Design review of the part built by this model. Coordinates are the model's own, in mm. A direction names the side the tool comes from. Coordinates: 2 decimals unless noted, no trailing zeros. Loops run counter-clockwise (first coordinate to the right, second up) from the corner with the lowest first, then second, coordinate; pieces in that order, holes last. Notation, with made-up numbers: M -31.5,54.25 L -19.5,54.25 A25 cw -19.5,77.25 Z; hole C 4.5,-23.5 d8. An arc over 180 degrees is marked long. Answer as a JSON object with one key per item and string values. Group by question number.
1. Consider section D-D (x = 10.5). State the section outline as (y, z) points.
2. Consider section A-A (x = -19). State the section outline as (y, z) points.
3. Insertion check: pin 1 (3 mm diameter, centred on x = 11.5, z = 9, fed in from -Y); pin 2 (6.5 mm diameter, centred on x = -10.5, z = 0, fed in from -Y); pin 3 (8.5 mm diameter, centred on x = 6, z = 0, fed in from +Y). Each pin has a flat end and moves straight along its axis. Give the tip position at first contact, or say it passes through.
4. To check wall thickness, follow probe 1 along Z at (x, y) = (0, 2); probe 2 along X at (y, z) = (15.5, 0); probe 3 along Y at (x, z) = (12, -17). State the ranges of each line that lie inside material, in increasing order.
5. Consider section B-B (z = -10.5). State the section outline as (x, y) points, then the cut area to 3 significant figures.
6. Consider section C-C (y = -5). State the section outline as (x, z) points, then the cut area to 3 significant figures.
7. Draft analysis for pull direction Z (two halves, no side actions). For faces 1 (the flat face through (3, 13, -1)), 2 (the cylindrical face through (21.477, 2.028, 4.769)), 3 (the flat face through (16.2, 4, 8.3)), state which applies: +Z half, -Z half, draft (parallel to the pull), parting line (faces both ways), or undercut.
8. Machinability: for faces 4 (the cylindrical face through (2.681, 11.521, -6.466)), 5 (the flat face through (3, 6, 9)), 6 (the cylindrical face through (21.477, 15.028, 4.769)), 7 (the flat face through (-0.3, 17, -14.4)), 8 (the flat face through (16.2, 13, -8.3)), which of the approach directions +Z, -Z, +X, -X, +Y, -Y give a long, thin tool a straight path to every point of the face, cutting with its end or side? Answer none if there is none.
from build123d import *

# Parameters (mm, degrees)
F3_R     = 1.965614
F4_DEPTH = 11.001
F5_R     = 1.5


with BuildPart() as f1:
    # F0 (on Right) → F1 (revolve)
    with BuildSketch(Plane.YZ):
        Polygon((13, -3), (-10, -3), (-10, -7), (6, -7), (6, -13.950632), (0, -13.950632), (0, -22), (4, -22), (4, -18), (13, -18), (13, -22), (17, -22), (17, -14), (10, -14), (10, -7), (13, -7), align=None)
    revolve(axis=Axis((0, -0.087436, 0), (0, 1, 0)))

    # F3 (on face) → F4 (cut, through all)
    with BuildSketch(Plane.XZ.offset(-6)):
        with Locations((10.5, 0)):
            Circle(F3_R)
        with Locations((7.424621, 7.424621)):
            Circle(F3_R)
        with Locations((0, 10.5)):
            Circle(F3_R)
        with Locations((-7.424621, 7.424621)):
            Circle(F3_R)
        with Locations((-10.5, 0)):
            Circle(F3_R)
        with Locations((-7.424621, -7.424621)):
            Circle(F3_R)
        with Locations((0, -10.5)):
            Circle(F3_R)
        with Locations((7.424621, -7.424621)):
            Circle(F3_R)
    extrude(amount=-F4_DEPTH, mode=Mode.SUBTRACT)

    # F5
    f5_edges = [f1.edges().sort_by_distance(p)[0] for p in [
        (0, 6, 7),
    ]]
    fillet(f5_edges, radius=F5_R)


solid = f1.part
Findings below:
{
 "1": {"outline": "M 0,-19.33 L 4,-19.33 L 4,-14.62 L 13,-14.62 L 13,-19.33 L 17,-19.33 L 17,-9.26 L 10,-9.26 L 10,-1.97 L 6,-1.97 L 6,-9.19 L 0,-9.19 Z; M 0,9.19 L 6,9.19 L 6,1.97 L 10,1.97 L 10,9.26 L 17,9.26 L 17,19.33 L 13,19.33 L 13,14.62 L 4,14.62 L 4,19.33 L 0,19.33 Z"},
 "2": {"outline": "M 0,-11.09 L 4,-11.09 L 4,11.09 L 0,11.09 Z; M 13,-11.09 L 17,-11.09 L 17,11.09 L 13,11.09 Z"},
 "3": {"pin 1": "stops at y = 0", "pin 2": "stops at y = 5.33", "pin 3": "stops at y = 13"},
 "4": {"probe 1": "z = -22 to -13.95, -7 to -3, 3 to 7, 13.95 to 22", "probe 2": "x = -22 to -14, 14 to 22", "probe 3": "y = 0 to 4, 13 to 17"},
 "5": {"outline": "M -19.33,0 L -9.19,0 L -9.19,6 L -1.97,6 L -1.97,10 L -9.26,10 L -9.26,17 L -19.33,17 L -19.33,13 L -14.62,13 L -14.62,4 L -19.33,4 Z; M 1.97,6 L 9.19,6 L 9.19,0 L 19.33,0 L 19.33,4 L 14.62,4 L 14.62,13 L 19.33,13 L 19.33,17 L 9.26,17 L 9.26,10 L 1.97,10 Z", "area": "317 mm^2"},
 "6": {"outline": "C 0,0 d14; hole C 0,0 d6", "area": "126 mm^2"},
 "7": {"face 1": "undercut", "face 2": "parting line", "face 3": "draft"},
 "8": {"face 4": "+Y", "face 5": "-Y", "face 6": "+Y, -Y", "face 7": "+Z, -Z, +X, -X, +Y", "face 8": "none"}
}
